Read the model definition and answer for the solid it produces. Units are mm, in the model's axes. A direction names the side the tool comes from. Coordinates: 2 decimals unless noted, no trailing zeros. Order: outer loops, then holes, each group sorted by start corner. A loop starts at its lowest first (then second) coordinate and runs counter-clockwise, first axis right, second up. Notation, with made-up numbers: (-27, 87.25) -> (-3, 87.25) arc R17 ccw to (-3, 108.25) -> close; hole circle Ø2 at (78.5, -18.5). An arc over 180 degrees is marked (long way). Use CSV: the item, a comma, the result in double quotes.
```python
from build123d import *

# Parameters (mm, degrees)
SKETCH1_W           = 14
SKETCH1_H           = 14.2
BOSS_EXTRUDE1_DEPTH = 3
SKETCH2_W           = 3
SKETCH2_H           = 3
SKETCH2_H_2         = 0.2
CUT_EXTRUDE1_DEPTH  = 10
SKETCH4_W           = 3
SKETCH4_H           = 3
SKETCH4_H_2         = 0.2
CUT_EXTRUDE2_DEPTH  = 10


with BuildPart() as part:
    # Sketch1 → Boss-Extrude1 (new body)
    with BuildSketch(Plane.XY):
        Rectangle(SKETCH1_W, SKETCH1_H)
    extrude(amount=BOSS_EXTRUDE1_DEPTH)

    # Sketch2 → Cut-Extrude1 (cut)
    with BuildSketch(Plane.XY.offset(3)):
        with Locations((-5.5, 5.6)):
            Rectangle(SKETCH2_W, SKETCH2_H)
        with Locations((-5.5, -1.4)):
            Rectangle(SKETCH2_W, SKETCH2_H)
        with Locations((-5.5, -7)):
            Rectangle(SKETCH2_W, SKETCH2_H_2)
    extrude(amount=-CUT_EXTRUDE1_DEPTH, mode=Mode.SUBTRACT)

    # Sketch4 → Cut-Extrude2 (cut)
    with BuildSketch(Plane.XY.offset(3)):
        with Locations((5.5, 5.6)):
            Rectangle(SKETCH4_W, SKETCH4_H)
        with Locations((5.5, -1.4)):
            Rectangle(SKETCH4_W, SKETCH4_H)
        with Locations((5.5, -7)):
            Rectangle(SKETCH4_W, SKETCH4_H_2)
    extrude(amount=-CUT_EXTRUDE2_DEPTH, mode=Mode.SUBTRACT)


solid = part.part
```
Item 1: The mould has two halves that part along Y. Classify faces 4 (the flat face through (-6, -2.9, 2)), 5 (the flat face through (5, 4.1, 2)), 6 (the flat face through (7, -5, 1)), 7 (the flat face through (0, -7.1, 1)): +Y half, -Y half, draft (parallel to the pull), parting line (faces both ways), or undercut.
Return value:
face 4,"undercut"
face 5,"+Y half"
face 6,"draft"
face 7,"-Y half"
Item 2: Find section C-C, the plane y = 5.75. Give the vertices of the cut face in (x, z).
Return value:
outline,"(-4, 0) -> (4, 0) -> (4, 3) -> (-4, 3) -> close"
Item 3: A tool of negligible diameter and unlimited length cuts with its end or side. For faces 1 (the flat face through (-4, -1, 2)), 2 (the flat face through (5, -2.9, 2)), 3 (the flat face through (-4, 6, 2)), from which of +Z, -Z, +X, -X, +Y, -Y can it reach the whole face along a straight path? Write none if from no direction.
Return value:
face 1,"+Z, -Z, -X"
face 2,"+Z, -Z, +X"
face 3,"+Z, -Z, -X, +Y"
Item 4: Each of these flat-tipped pins is pushed along its axis until it touches: P1, Ø0.9, axis at y = -1.5, z = 1, coming from the +X side; P2, Ø0.9, axis at x = 5.5, z = 1.5, coming from the +Y side; P3, Ø1.5, axis at y = 5, z = 2, coming from the -X side. Where does it stop, or does it pass through?
Return value:
P1,"stops at x = 4"
P2,"stops at y = 4.1"
P3,"stops at x = -4"
Item 5: Straight lines are drawn through the part: line 1 along Y through (x, z) = (5.5, 1.8); line 2 along X through (y, z) = (-1.75, 1.85). For each, find the intervals that lie inside material, in ascending order.
Return value:
line 1,"y = -6.9 to -2.9, 0.1 to 4.1"
line 2,"x = -4 to 4"
Item 6: Find section A-A, the plane x = -5.75. Give the vertices of the cut face in (y, z).
Return value:
outline,"(-6.9, 0) -> (-2.9, 0) -> (-2.9, 3) -> (-6.9, 3) -> close; (0.1, 0) -> (4.1, 0) -> (4.1, 3) -> (0.1, 3) -> close"
Item 7: Find section B-B, the plane z = 0.75. Give the vertices of the cut face in (x, y).
Return value:
outline,"(-7, -6.9) -> (-4, -6.9) -> (-4, -7.1) -> (4, -7.1) -> (4, -6.9) -> (7, -6.9) -> (7, -2.9) -> (4, -2.9) -> (4, 0.1) -> (7, 0.1) -> (7, 4.1) -> (4, 4.1) -> (4, 7.1) -> (-4, 7.1) -> (-4, 4.1) -> (-7, 4.1) -> (-7, 0.1) -> (-4, 0.1) -> (-4, -2.9) -> (-7, -2.9) -> close"
